Here's how the part is built. I have some questions about the finished solid (model axes, mm). A direction names the side the tool comes from. Round coordinates to 2 decimals unless told otherwise and drop trailing zeros. Write each loop counter-clockwise with the first axis right and the second up, starting at its lowest first coordinate (ties: lowest second). Pieces come first, ordered by that corner, then holes. Notation, with made-up numbers: (71, 3.25) - (83, 3.25) arc R23 cw to (83, 30.25) - close; hole circle Ø7 at (27.25, 69.5). An arc over 180 degrees is marked (long way). Write item = value, one per line. Start each with the question number.
Item 1: If we section it at A-A (y = 0): Please give me the cut outline in (x, z).
Item 2: Thinking about a two-plate mould opening in Z: for faces 4 (the face through (17.63, -2.93, -13.18)), 5 (the face through (11, 3.2, -8.1)), 6 (the face through (27, -11, 3)), which applies, pulls with the +Z half, pulls with the -Z half, needs draft (parallel to the pull), parting line crosses it, or undercut?
Item 3: For P1, Ø15.5, axis at y = 0, z = 0, coming from the +X side; P2, Ø1.5, axis at x = 17.5, y = -4, coming from the +Z side; P3, Ø6.5, axis at y = 3, z = -5, coming from the +X side; P4, Ø8, axis at x = 7, z = -4, coming from the -Y side, each with a flat end and sliding along its axis, tell me the tip position at first contact or that it passes through.
Item 4: Which directions (+Z, -Z, +X, -X, +Y, -Y) give clear straight access to the entire face, cutting with the end or side of a thin tool? Please do faces 1 (the face through (5.423, 4.57, -7.167)), 2 (the face through (18.89, -2.38, 10.74)), 3 (the face through (4.3, 10, 3.2)).
Item 5: If we section it at D-D (x = 17.5): Please give me the cut outline in (y, z), and give its area (3 significant figures).
Item 6: If I drill on line 1 along Z through (x, y) = (23.5, 0); line 2 along Z through (x, y) = (5.75, 0); line 3 along X through (y, z) = (-5, -8.5), over which ranges is the centre line in solid material (lowest first)? Write a range as [from, to].
Item 7: If we section it at C-C (x = 4.5): Please give me the cut outline in (y, z), and give its area (3 significant figures).
Autodesk Inventor part; units mm, degrees
ref_plane "YZ Plane" through (0, 0, 0) normal (1, 0, 0) x (0, 1, 0)
ref_plane "XZ Plane" through (0, 0, 0) normal (0, 1, 0) x (-1, 0, 0)
ref_plane "XY Plane" through (0, 0, 0) normal (0, 0, 1) x (1, 0, 0)
sketch "Sketch1" plane through (0, 0, 0) normal (0, 0, 1) x (1, 0, 0)
  line L0 (0, 0) -> (5, 0)
  line L1 (0, 8.5) -> (0, 10.5)
  line L2 (0, 10.5) -> (8, 10.5)
  line L3 (8, 10.5) -> (8, 13.5)
  line L4 (8, 13.5) -> (27, 13.5)
  line L5 (27, 13.5) -> (27, 11)
  line L6 (27, 11) -> (11, 11)
  line L7 (11, 11) -> (11, 8.5)
  line L8 (11, 8.5) -> (0, 8.5)
  dimension "d0" = 5
  dimension "d1" = 8.5
  dimension "d2" = 2
  dimension "d3" = 8
  dimension "d4" = 3
  dimension "d5" = 19
  dimension "d6" = 2.5
  dimension "d7" = 16
  dimension "d8" = 11
  dimension "d15" = 3
revolve "Revolution1" add sketch "Sketch1" angle 360 about axis through (0, 0, 0) along (1, 0, 0)
chamfer "Chamfer1" distance 0.5 angle 45 3 edges at (27, -13.5, 0) (8, -13.5, 0) (0, -10.5, 0)
thread "Thread1"
properties part number "logement roue libre"
Reply:
q1.outline = (0, -10) - (0.5, -10.5) - (8, -10.5) - (8, -13) - (8.5, -13.5) - (26.5, -13.5) - (27, -13) - (27, -11) - (11, -11) - (11, -8.5) - (0, -8.5) - close; (0, 8.5) - (11, 8.5) - (11, 11) - (27, 11) - (27, 13) - (26.5, 13.5) - (8.5, 13.5) - (8, 13) - (8, 10.5) - (0.5, 10.5) - (0, 10) - close
q2.face_4 = parting line crosses it
q2.face_5 = undercut
q2.face_6 = needs draft
q3.P1 = through
q3.P2 = 13.1
q3.P3 = 11
q3.P4 = -13.5
q4.face_1 = +X, -X
q4.face_2 = +X
q4.face_3 = -X
q5.outline = circle Ø27 at (0, 0); hole circle Ø22 at (0, 0)
q5.area = 192 mm2
q6.line_1 = [-13.5, -11], [11, 13.5]
q6.line_2 = [-10.5, -8.5], [8.5, 10.5]
q6.line_3 = [0, 11]
q7.outline = circle Ø21 at (0, 0); hole circle Ø17 at (0, 0)
q7.area = 119 mm2
